Check sheet for the modelled part. Datum: model origin and axes. Units: mm. Face numbers are marked on the shaded views. A direction names the side the tool comes from. Give positions to 0.01 mm unless a question says otherwise; leave off trailing zeros. Loops run counter-clockwise (first coordinate to the right, second up) from the corner with the lowest first, then second, coordinate; pieces in that order, holes last. Notation, with made-up numbers: M 47.5,-17 L 77.5,-17 A18 ccw 77.5,-10 Z; hole C 68,65.5 d10. An arc over 180 degrees is marked long. Write each question's results on one line, items separated by ' | '. Start each with the question number.
1. Sectioned sample at C-C on y = 15.5. Record the cut outline in (x, z).
2. Sectioned sample at D-D on z = 19. Record the cut outline in (x, y).
3. Go/stop test with flat-tipped pins: pin 1 (6 mm diameter, centred on x = -14.5, z = 52.5, fed in from -Y); pin 2 (3 mm diameter, centred on y = -40, z = 37.5, fed in from -X); pin 3 (1.5 mm diameter, centred on x = -7.5, z = 12, fed in from -Y). Record where each tip stops, or that it passes through.
4. Sectioned sample at A-A on x = 0. Record the cut outline in (y, z).
5. Tool access check on the marked faces 4, 5, 6, 7 and 8. Record the directions out of +Z, -Z, +X, -X, +Y, -Y that give a thin tool (end or side, any length) a straight path to the whole face; none if there is none.
6. Sectioned sample at B-B on y = 0. Record the cut outline in (x, z).
7. Draft check along Z on the marked faces 1, 2 and 3. Enter one of: pulls with the +Z half, pulls with the -Z half, needs draft (parallel to the pull), parting line crosses it, or undercut.
8. Material ranges on line 1 along Z through (x, y) = (-0.5, 0); line 2 along Y through (x, z) = (-5, 27); line 3 along Z through (x, y) = (13, -16.5), recorded low to high.
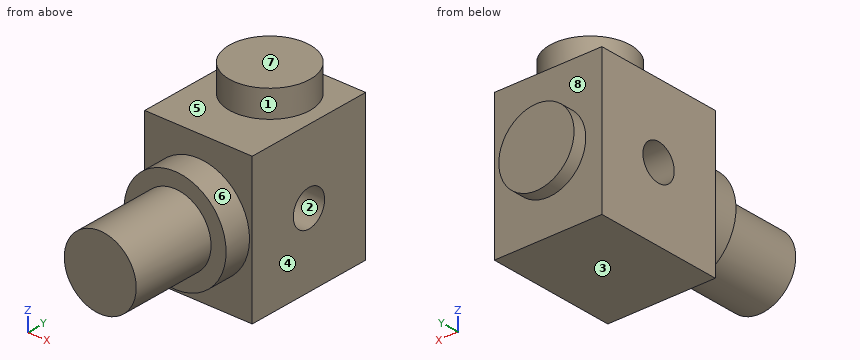
```python
from build123d import *

# Parameters (mm, degrees)
SKETCH1_W           = 48.5
SKETCH1_H           = 40
BOSS_EXTRUDE1_DEPTH = 54
SKETCH2_R           = 15
BOSS_EXTRUDE2_DEPTH = 10
SKETCH3_R           = 14
BOSS_EXTRUDE3_DEPTH = 5
SKETCH4_R           = 19
BOSS_EXTRUDE4_DEPTH = 10
SKETCH5_R           = 13.38588386
BOSS_EXTRUDE5_DEPTH = 32
SKETCH6_R           = 6.7
CUT_EXTRUDE1_DEPTH  = 20
SKETCH7_R           = 6.7
CUT_EXTRUDE2_DEPTH  = 20


with BuildPart() as part:
    # Sketch1 → Boss-Extrude1 (new body)
    with BuildSketch(Plane(origin=(0, 0, 0), x_dir=(0, 1, 0), z_dir=(0, 0, 1))):
        Rectangle(SKETCH1_W, SKETCH1_H)
    extrude(amount=BOSS_EXTRUDE1_DEPTH)

    # Sketch2 → Boss-Extrude2 (add)
    with BuildSketch(Plane.XY.offset(54)):
        with Locations((0, 6.25)):
            Circle(SKETCH2_R)
    extrude(amount=BOSS_EXTRUDE2_DEPTH)

    # Sketch3 → Boss-Extrude3 (add)
    with BuildSketch(Plane(origin=(0, 24.25, 0), x_dir=(-1, 0, 0), z_dir=(0, 1, 0))):
        with Locations((0, 26.873266577)):
            Circle(SKETCH3_R)
    extrude(amount=BOSS_EXTRUDE3_DEPTH)

    # Sketch4 → Boss-Extrude4 (add)
    with BuildSketch(Plane.XZ.offset(24.25)):
        with Locations((0, 27)):
            Circle(SKETCH4_R)
    extrude(amount=BOSS_EXTRUDE4_DEPTH)

    # Sketch5 → Boss-Extrude5 (add)
    with BuildSketch(Plane.XZ.offset(34.25)):
        with Locations((0, 27)):
            Circle(SKETCH5_R)
    extrude(amount=BOSS_EXTRUDE5_DEPTH)

    # Sketch6 → Cut-Extrude1 (cut)
    with BuildSketch(Plane.YZ.offset(20)):
        with Locations((0, 27)):
            Circle(SKETCH6_R)
    extrude(amount=-CUT_EXTRUDE1_DEPTH, mode=Mode.SUBTRACT)

    # Sketch7 → Cut-Extrude2 (cut)
    with BuildSketch(Plane(origin=(-20, 0, 0), x_dir=(0, -1, 0), z_dir=(-1, 0, 0))):
        with Locations((0, 27)):
            Circle(SKETCH7_R)
    extrude(amount=-CUT_EXTRUDE2_DEPTH, mode=Mode.SUBTRACT)


solid = part.part
```
Output values:
1) outline: M -20,0 L 20,0 L 20,54 L 11.81,54 L 11.81,64 L -11.81,64 L -11.81,54 L -20,54 Z
2) outline: M -20,-24.25 L -17.23,-24.25 L -17.23,-34.25 L -10.73,-34.25 L -10.73,-66.25 L 10.73,-66.25 L 10.73,-34.25 L 17.23,-34.25 L 17.23,-24.25 L 20,-24.25 L 20,24.25 L 11.58,24.25 L 11.58,29.25 L -11.58,29.25 L -11.58,24.25 L -20,24.25 Z
3) pin 1: y = -24.25 | pin 2: x = -9.91 | pin 3: y = -34.25
4) outline: M -66.25,13.61 L -34.25,13.61 L -34.25,8 L -24.25,8 L -24.25,0 L 24.25,0 L 24.25,12.87 L 29.25,12.87 L 29.25,40.87 L 24.25,40.87 L 24.25,54 L 21.25,54 L 21.25,64 L -8.75,64 L -8.75,54 L -24.25,54 L -24.25,46 L -34.25,46 L -34.25,40.39 L -66.25,40.39 Z; hole C 0,27 d13.4
5) face 4: +Z, -Z, +X, +Y, -Y | face 5: +Z | face 6: -Y | face 7: +Z, +X, -X, +Y, -Y | face 8: +Y
6) outline: M -20,0 L 20,0 L 20,20.3 L -20,20.3 Z; M -20,33.7 L 20,33.7 L 20,54 L 13.64,54 L 13.64,64 L -13.64,64 L -13.64,54 L -20,54 Z
7) face 1: needs draft | face 2: undercut | face 3: pulls with the -Z half
8) line 1: 0 to 20.3, 33.7 to 64 | line 2: -66.25 to -6.7, 6.7 to 29.25 | line 3: 0 to 54
